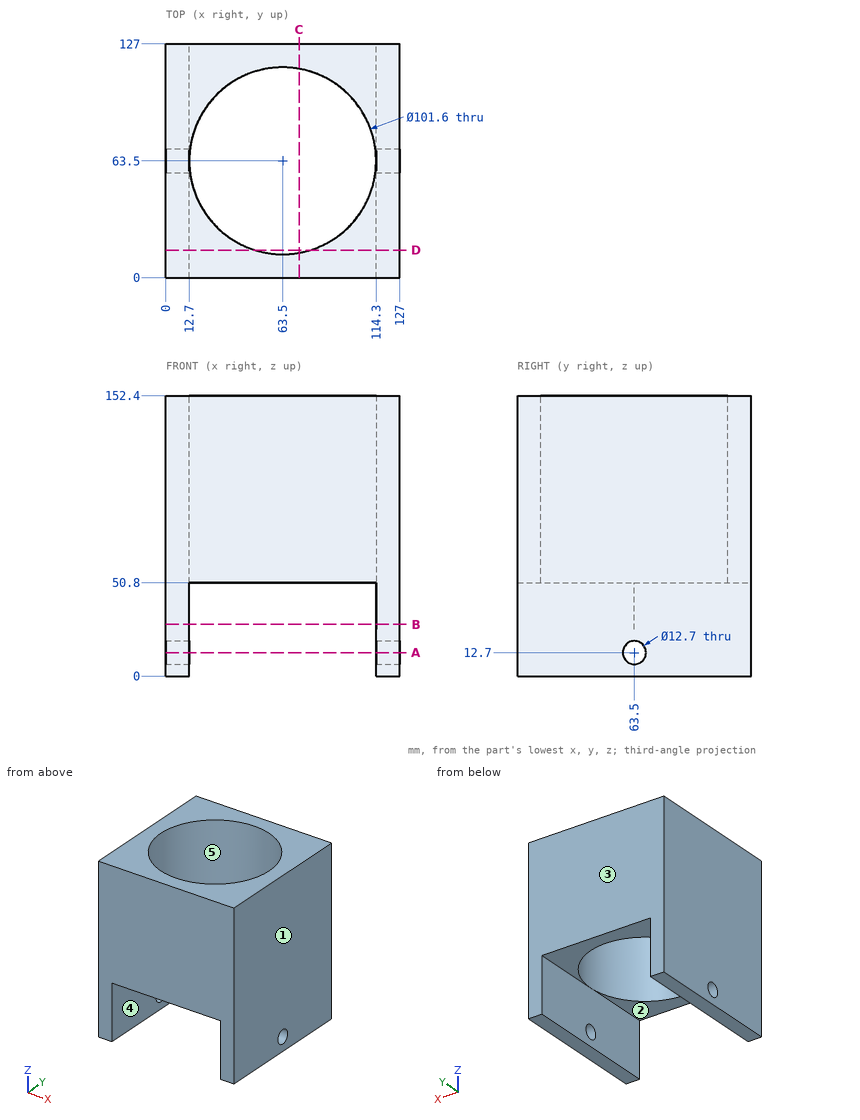
Part print with two shaded views. Sizes in mm from the minimum x, y, z corner. A direction names the side the tool comes from. Coordinates: 2 decimals unless noted, no trailing zeros. Write each loop counter-clockwise with the first axis right and the second up, starting at its lowest first coordinate (ties: lowest second). Pieces come first, ordered by that corner, then holes.
(1) Cut at D-D on y = 15. List the corners of the cut face in (x, z), and give its area (3 significant figures).
(2) Cut at C-C on x = 72.5. List the corners of the cut face in (y, z), and give its area (3 significant figures).
(3) Cut at B-B on z = 28. List the corners of the cut face in (x, y), and give its area (3 significant figures).
(4) Cut at A-A on z = 12.7. List the corners of the cut face in (x, y), and give its area (3 significant figures).
(5) 3-axis set-ups, long thin cutter, end or side, ignore diameter. For the marked faces 1 and 2: which of +Z, -Z, +X, -X, +Y, -Y reach the whole face in a straight line?
(6) Pin check, flat tips, straight feed: pin 1 Ø4 at (x, z) = (35, 136) entering from -Y; pin 2 Ø2 at (x, y) = (35.5, 15) entering from -Z. Stop position of each tip, or through.
(7) Mould opens along Y. For the marked faces 3, 4 and 5 say: pulls with the +Y half, pulls with the -Y half, needs draft (parallel to the pull), parting line crosses it, or undercut.
(8) Drill centre lines: line 1 (X direction, y = 11.5, z = 24.5); line 2 (Z direction, x = 6.25, y = 63.5). Where is each one in solid material? Low to high.
Working result:
1. outline: (0, 0) - (12.7, 0) - (12.7, 50.8) - (48.39, 50.8) - (48.39, 152.4) - (0, 152.4) - close; (78.61, 50.8) - (114.3, 50.8) - (114.3, 0) - (127, 0) - (127, 152.4) - (78.61, 152.4) - close
1. area: 11,100 mm2
2. outline: (0, 50.8) - (13.5, 50.8) - (13.5, 152.4) - (0, 152.4) - close; (113.5, 50.8) - (127, 50.8) - (127, 152.4) - (113.5, 152.4) - close
2. area: 2,740 mm2
3. outline: (0, 0) - (12.7, 0) - (12.7, 127) - (0, 127) - close; (114.3, 0) - (127, 0) - (127, 127) - (114.3, 127) - close
3. area: 3,230 mm2
4. outline: (0, 0) - (12.7, 0) - (12.7, 57.15) - (0, 57.15) - close; (0, 69.85) - (12.7, 69.85) - (12.7, 127) - (0, 127) - close; (114.3, 0) - (127, 0) - (127, 57.15) - (114.3, 57.15) - close; (114.3, 69.85) - (127, 69.85) - (127, 127) - (114.3, 127) - close
4. area: 2,900 mm2
5. face 1: +Z, -Z, +X, +Y, -Y
5. face 2: -Z, +Y, -Y
6. pin 1: stops at y = 0
6. pin 2: stops at z = 50.8
7. face 3: pulls with the +Y half
7. face 4: needs draft
7. face 5: undercut
8. line 1: x = 0 to 12.7, 114.3 to 127
8. line 2: z = 0 to 6.35, 19.05 to 152.4
